Model file for the job. Use its own axes, mm. A direction names the side the tool comes from. Coordinates: 2 decimals unless noted, no trailing zeros. Loops run counter-clockwise (first coordinate to the right, second up) from the corner with the lowest first, then second, coordinate; pieces in that order, holes last.
Autodesk Inventor part; units mm, degrees
ref_plane "YZ Plane" through (0, 0, 0) normal (1, 0, 0) x (0, 1, 0)
ref_plane "XZ Plane" through (0, 0, 0) normal (0, 1, 0) x (-1, 0, 0)
ref_plane "XY Plane" through (0, 0, 0) normal (0, 0, 1) x (1, 0, 0)
sketch "草图1" plane through (0, 0, 0) normal (0, 0, 1) x (1, 0, 0)
  circle A0 centre (0, 39.5) radius 25
  line L0 (-25, 46.1987) -> (-25, 0)
  line L1 (-25, 0) -> (25, 0)
  line L2 (25, 0) -> (25, 46.1987)
  line L3 (-21.6506, 52) -> (-51.6728, 0)
  line L4 (21.6506, 52) -> (51.6728, 0)
  line L5 (0, 0) -> (0, -13.7014)
  dimension "d0" = 50
  dimension "d1" = 39.5
  dimension "d2" = 13.7014
  dimension "d3" = 60
extrude "拉伸1" add sketch "草图1" along normal blind 5
sketch "草图2" plane through (0, 0, 5) normal (0, 0, 1) x (1, 0, 0)
  circle A0 centre (0, 39.5) radius 16
  circle A1 centre (0, 39.5) radius 11
  arc A2 (21.6506, 52) -> (-21.6506, 52) centre (0, 39.5) ccw
  point P0 (0, 0)
  dimension "d6" = 32
  dimension "d7" = 22
extrude "拉伸2" add sketch "草图2" along normal blind 4
sketch "草图3" plane through (0, 39.5, 9) normal (0, 0, 1) x (1, 0, 0)
  circle A0 centre (0, 0) radius 16
  circle A1 centre (0, 0) radius 15
  circle A2 centre (0, 0) radius 11
  point P0 (0, -39.5)
  dimension "d10" = 32
  dimension "d11" = 30
extrude "拉伸3" cut sketch "草图3" against normal blind 1.5 contours A0
sketch "草图4" plane through (0, 39.5, 5) normal (0, 0, 1) x (1, 0, 0)
  circle A0 centre (0, 0) radius 7.5
  circle A1 centre (0, 0) radius 11
  point P0 (0, -39.5)
  dimension "d14" = 15
extrude "拉伸4" cut sketch "草图4" against normal through all contours A0
sketch "草图5" plane through (0, 0, 5) normal (0, 0, 1) x (1, 0, 0)
  circle A0 centre (15, 10) radius 2
  circle A1 centre (-15, 10) radius 2
  circle A2 centre (15, 53.4732) radius 2
  circle A3 centre (-15, 53.4732) radius 2
  line L0 (25, 0) -> (25, 46.1987)
  line L1 (-25, 0) -> (25, 0)
  line L2 (-25, 46.1987) -> (-25, 0)
  arc A4 (15, 53.4732) -> (-15, 53.4732) centre (0, 39.5) ccw
  circle A5 centre (0, 39.5) radius 7.5
  point P0 (0, 0)
  dimension "d17" = 4
  dimension "d18" = 4
  dimension "d19" = 4
  dimension "d20" = 4
  dimension "d21" = 10
  dimension "d22" = 10
  dimension "d23" = 10
  dimension "d24" = 10
  dimension "d25" = 20.5
  dimension "d26" = 10
  dimension "d27" = 10
extrude "拉伸5" add sketch "草图5" along normal blind 18 contours A0 | A1 | A2 | A3
thread "螺纹1"
thread "螺纹2"
thread "螺纹3"
thread "螺纹4"
chamfer "倒角1" distance 0.25 angle 45 4 edges at (-17, 53.4732, 23) (13, 53.4732, 23) (13, 10, 23) (-17, 10, 23)
properties part number "刀轴端盖"
Q1. Slice it at B-B (z = 6.5). List the corners of the cut face in (x, y).
Answers:
outline: circle Ø4 at (-15, 10); circle Ø4 at (-15, 53.47); circle Ø32 at (0, 39.5); circle Ø4 at (15, 10); circle Ø4 at (15, 53.47); hole circle Ø22 at (0, 39.5)
Q2. Drill centre lines: line 1 (Z direction, x = 12.5, y = 13); line 2 (Z direction, x = 15, y = 42.5); line 3 (Y direction, x = -8, z = 6.5). Where is each one in solid material? Low to high.
Answers:
line 1: z = 0 to 5
line 2: z = 0 to 7.5
line 3: y = 25.64 to 31.95, 47.05 to 53.36
Q3. Mould opens along X. For faces 3 (the flat face through (0, 26, 0)), 4 (the flat face through (-23.3, 49.14, 2.46)), 5 (the cylindrical face through (-0.367, 64.497, 2.465)), 6 (the cylindrical face through (14.566, 55.426, 13.751)) say: +X half, -X half, draft (parallel to the pull), parting line (faces both ways), or undercut.
Answers:
face 3: draft
face 4: -X half
face 5: parting line
face 6: undercut
Q4. Slice it at D-D (y = 42.5). List the corners of the cut face in (x, z).
Answers:
outline: (-25, 0) - (-6.87, 0) - (-6.87, 5) - (-10.58, 5) - (-10.58, 9) - (-14.7, 9) - (-14.7, 7.5) - (-15.72, 7.5) - (-15.72, 5) - (-25, 5) - close; (6.87, 0) - (25, 0) - (25, 5) - (15.72, 5) - (15.72, 7.5) - (14.7, 7.5) - (14.7, 9) - (10.58, 9) - (10.58, 5) - (6.87, 5) - close
Q5. Flat gauge pins, fed straight in: P1, Ø8, axis at x = -14.5, z = 4, coming from the +Y side; P2, Ø12, axis at x = 18.5, z = 13, coming from the +Y side; P3, Ø2, axis at y = 34, z = 10.5, coming from the -X side; P4, Ø5, axis at y = 7.5, z = 17, coming from the -X side. Where does each tip first touch, or does it go through?
Answers:
P1: stops at y = 62.19
P2: stops at y = 55.47
P3: passes through
P4: stops at x = -17
Q6. Which spindle directions (+Z, -Z, +X, -X, +Y, -Y) get a long thin tool onto all of the face, cutting with end or side? Do faces 1 (the flat face through (-5, 50, 9)), 2 (the flat face through (25, 23, 2)). Say none if no direction does.
Answers:
face 1: +Z
face 2: +Z, -Z, +X, +Y, -Y
Q7. Slice it at A-A (x = 0). List the corners of the cut face in (y, z), and give its area (4 significant figures).
Answers:
outline: (0, 0) - (32, 0) - (32, 5) - (28.5, 5) - (28.5, 9) - (24.5, 9) - (24.5, 7.5) - (23.5, 7.5) - (23.5, 5) - (0, 5) - close; (47, 0) - (64.5, 0) - (64.5, 5) - (55.5, 5) - (55.5, 7.5) - (54.5, 7.5) - (54.5, 9) - (50.5, 9) - (50.5, 5) - (47, 5) - close
area: 284.5 mm2
Q8. Slice it at C-C (y = 10). List the corners of the cut face in (x, z), and give its area (3 significant figures).
Answers:
outline: (-25, 0) - (25, 0) - (25, 5) - (17, 5) - (17, 22.75) - (16.75, 23) - (13.25, 23) - (13, 22.75) - (13, 5) - (-13, 5) - (-13, 22.75) - (-13.25, 23) - (-16.75, 23) - (-17, 22.75) - (-17, 5) - (-25, 5) - close
area: 394 mm2
